Geometry check sheet. Reference: drawing and pictorial views, mm from the part's lowest x, y, z. Give positions to 0.01 mm unless a question says otherwise; leave off trailing zeros. Write each loop counter-clockwise with the first axis right and the second up, starting at its lowest first coordinate (ties: lowest second). Pieces come first, ordered by that corner, then holes. Notation, with made-up numbers: (60, 38.25) -> (65, 38.25) arc R22 ccw to (65, 77.25) -> close; hole circle Ø11 at (-29.5, 26). An arc over 180 degrees is marked (long way). Use a Markdown table: item, result. Add a question column.
1. Scan lines: probe 1 along Y at (x, z) = (240, 2); probe 2 along X at (y, z) = (4, 1.4); probe 3 along X at (y, z) = (15, 0.4). Record each from-to range of solid material in increasing order. Write a range as [from, to].
2. Cross-section at B-B (z = 2.85). Enter the section's corners in (x, y), then the cut area to 3 significant figures.
3. Cross-section at A-A (x = 240). Enter the section's corners in (y, z), then the cut area to 3 significant figures.
4. Gauge pin test, flat ends, axial feed: P1, Ø2, axis at y = 15, z = 2.5, coming from the +X side; P2, Ø1.8, axis at x = 1.5, z = 2.5, coming from the -Y side; P3, Ø1.4, axis at y = 22, z = 3.5, coming from the -X side. Record the tip position at first contact, or that the pin passes through.
5. Cross-section at C-C (x = 208). Enter the section's corners in (y, z).
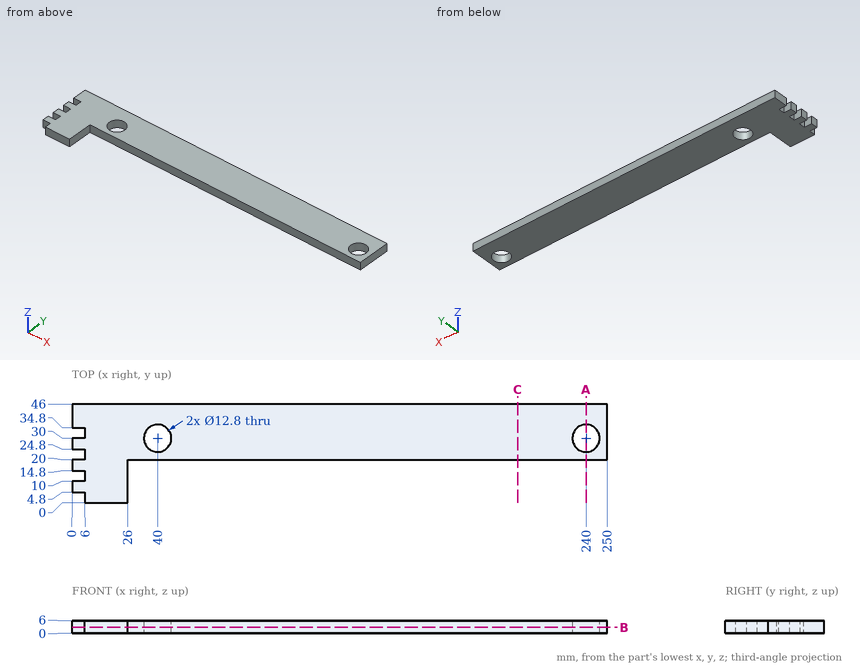
Worked answers:
| question | item | result |
|---|---|---|
| 1 | probe 1 | y = [20, 23.6], [36.4, 46] |
| 1 | probe 2 | x = [6, 26] |
| 1 | probe 3 | x = [0, 26] |
| 2 | outline | (0, 4.8) -> (6, 4.8) -> (6, 0) -> (26, 0) -> (26, 20) -> (250, 20) -> (250, 46) -> (0, 46) -> (0, 34.8) -> (6, 34.8) -> (6, 30) -> (0, 30) -> (0, 24.8) -> (6, 24.8) -> (6, 20) -> (0, 20) -> (0, 14.8) -> (6, 14.8) -> (6, 10) -> (0, 10) -> close; hole circle Ø12.8 at (40, 30); hole circle Ø12.8 at (240, 30) |
| 2 | area | 6,650 mm² |
| 3 | outline | (20, 0) -> (23.6, 0) -> (23.6, 6) -> (20, 6) -> close; (36.4, 0) -> (46, 0) -> (46, 6) -> (36.4, 6) -> close |
| 3 | area | 79.2 mm² |
| 4 | P1 | stops at x = 26 |
| 4 | P2 | stops at y = 4.8 |
| 4 | P3 | stops at x = 6 |
| 5 | outline | (20, 0) -> (46, 0) -> (46, 6) -> (20, 6) -> close |
